from build123d import *

# Parameters (mm, degrees)
BOSS_EXTRUDE1_DEPTH  = 15
FILLET1_R            = 1
SKETCH6_W            = 30
SKETCH6_H            = 38
CUT_EXTRUDE2_DEPTH   = 6.35
M4_CLEARANCE_HOLE1_D = 4.5
CUT_EXTRUDE3_START   = -5
SKETCH11_R           = 4.125
CUT_EXTRUDE3_DEPTH   = 40.35
M4_CLEARANCE_HOLE2_D = 4.5
CUT_EXTRUDE4_START   = -4
SKETCH15_R           = 4.125
CUT_EXTRUDE4_DEPTH   = 78.35
SKETCH16_W           = 22.054388556
SKETCH16_H           = 29.268630824
CUT_EXTRUDE6_DEPTH   = 8.25
SKETCH18_W           = 30
SKETCH18_H           = 5
BOSS_EXTRUDE2_DEPTH  = 3
CHAMFER1_SIZE        = 5
CHAMFER1_SIZE2       = 2.886751346


with BuildPart() as part:
    # Sketch2 → Boss-Extrude1 (new, symmetric)
    with BuildSketch(Plane(origin=(0, 0, 0), x_dir=(0, 0, -1), z_dir=(1, 0, 0))):
        Polygon((0, 5.65), (0, 80.65), (-50, 5.65), (-50, 0), (-50, -6.35), (48.05, -6.35), (48.05, 0), (28.05, 20), (28.05, 5.65), align=None)
    extrude(amount=BOSS_EXTRUDE1_DEPTH, both=True)

    # Fillet1
    fillet1_edges = [part.edges().sort_by_distance(p)[0] for p in [
        (0, 80.65, 0),
        (0, 20, -28.05),
    ]]
    fillet(fillet1_edges, radius=FILLET1_R)

    # Sketch6 → Cut-Extrude2 (cut)
    with BuildSketch(Plane.XZ.offset(6.35)):
        with Locations((0, 31)):
            Rectangle(SKETCH6_W, SKETCH6_H)
    extrude(amount=-CUT_EXTRUDE2_DEPTH, mode=Mode.SUBTRACT)

    # M4 Clearance Hole1 (through all)
    with Locations(Plane(origin=(0, 0, 0), x_dir=(-1, 0, 0), z_dir=(0, 0, -1))):
        with Locations((0, 58.347224362), (0, 40.847224362), (0, 23.347224362)):
            Hole(M4_CLEARANCE_HOLE1_D / 2)

    # Sketch11 → Cut-Extrude3 (cut)
    with BuildSketch(Plane(origin=(0, 0, 0), x_dir=(-1, 0, 0), z_dir=(0, 0, -1)).offset(CUT_EXTRUDE3_START)):
        with Locations((0, 58.347224362)):
            Circle(SKETCH11_R)
        with Locations((0, 40.847224362)):
            Circle(SKETCH11_R)
        with Locations((0, 23.347224362)):
            Circle(SKETCH11_R)
    extrude(amount=-CUT_EXTRUDE3_DEPTH, mode=Mode.SUBTRACT)

    # M4 Clearance Hole2 (through all)
    with Locations(Plane(origin=(0, 0, 0), x_dir=(-1, 0, 0), z_dir=(0, -1, 0))):
        with Locations((0, -37), (0, -22)):
            Hole(M4_CLEARANCE_HOLE2_D / 2)

    # Sketch15 → Cut-Extrude4 (cut)
    with BuildSketch(Plane.XZ.offset(CUT_EXTRUDE4_START)):
        with Locations(Location((0, 37, 0), (0, 0, 270))):
            Circle(SKETCH15_R)
        with Locations(Location((0, 22, 0), (0, 0, 270))):
            Circle(SKETCH15_R)
    extrude(amount=-CUT_EXTRUDE4_DEPTH, mode=Mode.SUBTRACT)

    # Sketch16 → Cut-Extrude6 (cut)
    with BuildSketch(Plane(origin=(-4.125, 0, 0), x_dir=(0, 0, -1), z_dir=(1, 0, 0))):
        with Locations((-33.027194278, 37.981539774)):
            Rectangle(SKETCH16_W, SKETCH16_H)
    extrude(amount=CUT_EXTRUDE6_DEPTH, mode=Mode.SUBTRACT)

    # Sketch18 → Boss-Extrude2 (add)
    with BuildSketch(Plane.XZ.offset(6.35)):
        with Locations((0, -50.55)):
            Rectangle(SKETCH18_W, SKETCH18_H)
    extrude(amount=-BOSS_EXTRUDE2_DEPTH)

    # Chamfer1
    chamfer1_edges = [part.edges().sort_by_distance(p)[0] for p in [
        (-15, -4.85, -53.05),
        (15, -4.85, -53.05),
    ]]
    chamfer1_side = [part.faces().sort_by_distance(p)[0] for p in [
        (0, -4.85, -53.05),
    ]]
    chamfer(chamfer1_edges, length=CHAMFER1_SIZE, length2=CHAMFER1_SIZE2, reference=chamfer1_side[0])


solid = part.part
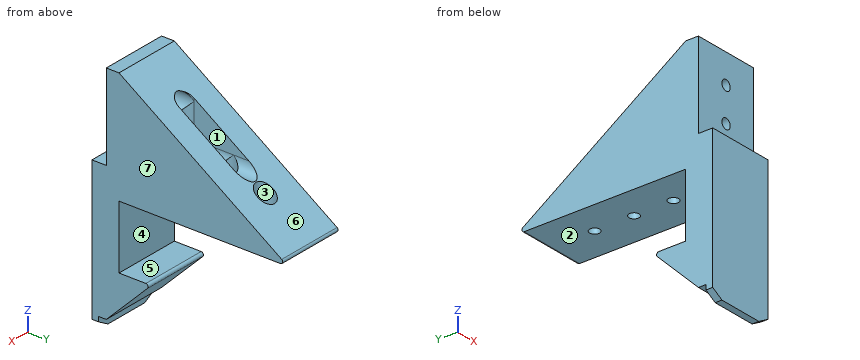
The model under review builds one solid part; all positions refer to its coordinate system, in mm. Face numbers are marked on the shaded views. A direction names the side the tool comes from. Coordinates: 2 decimals unless noted, no trailing zeros. Order: outer loops, then holes, each group sorted by start corner. A loop starts at its lowest first (then second) coordinate and runs counter-clockwise, first axis right, second up. Notation, with made-up numbers: (50, -19.5) -> (57, -19.5) arc R16 ccw to (57, -15.5) -> close; hole circle Ø8 at (41.5, 88.25). An arc over 180 degrees is marked (long way). Answer in a Markdown table with one row per item.
(1) Consider section B-B (x = -8.5). Write out the cut boundary in (y, z).
Answers:
| item | result |
|---|---|
| outline | (-6.35, -53.05) -> (-3.35, -53.05) -> (-3.35, -48.05) -> (0, -48.05) -> (18.29, -29.76) arc R1 ccw to (17.59, -28.05) -> (5.65, -28.05) -> (5.65, 0) -> (77.35, 0) arc R1 ccw to (77.9, 1.83) -> (5.65, 50) -> (0, 50) -> (0, 12) -> (-6.35, 12) -> close |
(2) Wall thickness on line 1 along Y through (x, z) = (0, 14); line 2 along Y through (x, z) = (0, 8.5); line 3 along X through (y, z) = (10, 37) (3 decimals): over which ranges is each line inside the solid? List them lowest first.
Answers:
| item | result |
|---|---|
| line 1 | 0 to 19.22, 27.47 to 36.72, 44.97 to 54.22 |
| line 2 | -6.35 to 19.22, 27.47 to 36.72, 44.97 to 54.22, 62.47 to 67.9 |
| line 3 | -15 to -4.125, 4.125 to 15 |
(3) Insertion check: pin 1 (4 mm diameter, centred on x = 0.5, z = -49.5, fed in from +Y); pin 2 (3 mm diameter, centred on x = -4.5, y = 43.5, fed in from -Z); pin 3 (1.7 mm diameter, centred on x = -3, y = -2, fed in from -Z). Each pin has a flat end and moves straight along its axis. Give the tip position at first contact, or say it passes through.
Answers:
| item | result |
|---|---|
| pin 1 | y = 0.55 |
| pin 2 | z = 0 |
| pin 3 | z = -48.05 |
(4) Consider section D-D (z = -34). Write out the cut boundary in (x, y), plus the area to 3 significant figures.
Answers:
| item | result |
|---|---|
| outline | (-15, -6.35) -> (15, -6.35) -> (15, 14.05) -> (-15, 14.05) -> close |
| area | 612 mm² |
(5) Machinability: for the marked faces 1, 2 and 3, which of the approach directions +Z, -Z, +X, -X, +Y, -Y give a long, thin tool a straight path to every point of the face, cutting with its end or side? Answer none if there is none.
Answers:
| item | result |
|---|---|
| face 1 | +Z, +Y |
| face 2 | +X, -X, +Y |
| face 3 | +Z |
(6) The part is to be moulded in two halves that separate along Z. For the marked faces 4, 5, 6 and 7, say which applies: +Z half, -Z half, draft (parallel to the pull), parting line (faces both ways), or undercut.
Answers:
| item | result |
|---|---|
| face 4 | undercut |
| face 5 | undercut |
| face 6 | +Z half |
| face 7 | draft |
(7) Consider section A-A (y = 10.5). Write out the cut boundary in (x, z) (3 decimals).
Answers:
| item | result |
|---|---|
| outline | (-15, -37.55) -> (15, -37.55) -> (15, -28.05) -> (-15, -28.05) -> close; (-15, 0) -> (15, 0) -> (15, 46.767) -> (-15, 46.767) -> close; hole circle Ø8.25 at (0, 22); hole circle Ø8.25 at (0, 37) |
(8) Consider section C-C (z = 10.5). Write out the cut boundary in (x, y) (3 decimals), plus the area to 3 significant figures.
Answers:
| item | result |
|---|---|
| outline | (-15, -6.35) -> (15, -6.35) -> (15, 64.9) -> (-15, 64.9) -> close; hole circle Ø8.25 at (0, 23.347); hole circle Ø8.25 at (0, 40.847); hole circle Ø8.25 at (0, 58.347) |
| area | 1,980 mm² |
